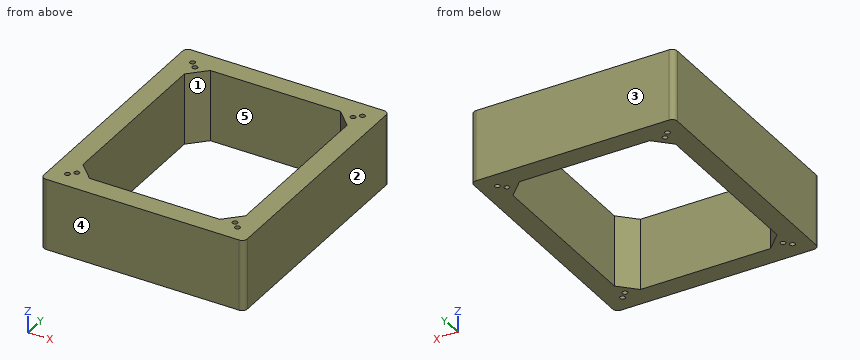
from build123d import *

# Parameters (mm, degrees)
F0_R     = 1.5875
F1_DEPTH = 44.45


with BuildPart() as f1:
    # F0 (on Top) → F1 (new body)
    with BuildSketch(Plane.XY):
        with BuildLine():
            Line((60.531797, 76.456334), (-60.118203, 76.456334))
            ThreePointArc((-60.118203, 76.456334), (-62.363267, 75.526399), (-63.293203, 73.281334))
            Line((-63.293203, 73.281334), (-63.293203, -72.768666))
            ThreePointArc((-63.293203, -72.768666), (-62.363267, -75.01373), (-60.118203, -75.943666))
            Line((-60.118203, -75.943666), (60.531797, -75.943666))
            ThreePointArc((60.531797, -75.943666), (62.776861, -75.01373), (63.706797, -72.768666))
            Line((63.706797, -72.768666), (63.706797, 73.281334))
            ThreePointArc((63.706797, 73.281334), (62.776861, 75.526399), (60.531797, 76.456334))
        make_face()
        with BuildLine():
            ThreePointArc((-56.943203, 66.931334), (-56.013267, 69.176399), (-53.768203, 70.106334))
            Line((-53.768203, 70.106334), (54.181797, 70.106334))
            ThreePointArc((54.181797, 70.106334), (56.426861, 69.176399), (57.356797, 66.931334))
            Line((57.356797, 66.931334), (57.356797, -66.418666))
            ThreePointArc((57.356797, -66.418666), (56.426861, -68.66373), (54.181797, -69.593666))
            Line((54.181797, -69.593666), (-53.768203, -69.593666))
            ThreePointArc((-53.768203, -69.593666), (-56.013267, -68.66373), (-56.943203, -66.418666))
            Line((-56.943203, -66.418666), (-56.943203, 66.931334))
        make_face(mode=Mode.SUBTRACT)
        with BuildLine():
            Line((54.181797, 70.106334), (-53.768203, 70.106334))
            ThreePointArc((-53.768203, 70.106334), (-56.013267, 69.176399), (-56.943203, 66.931334))
            Line((-56.943203, 66.931334), (-56.943203, -66.418666))
            ThreePointArc((-56.943203, -66.418666), (-56.013267, -68.66373), (-53.768203, -69.593666))
            Line((-53.768203, -69.593666), (54.181797, -69.593666))
            ThreePointArc((54.181797, -69.593666), (56.426861, -68.66373), (57.356797, -66.418666))
            Line((57.356797, -66.418666), (57.356797, 66.931334))
            ThreePointArc((57.356797, 66.931334), (56.426861, 69.176399), (54.181797, 70.106334))
        make_face()
        with Locations((-52.834257, -65.484719)):
            Circle(F0_R, mode=Mode.SUBTRACT)
        with BuildLine():
            ThreePointArc((-48.268948, 63.640233), (-47.847518, 63.727175), (-47.418203, 63.756334))
            Line((-47.418203, 63.756334), (-40.433203, 63.756334))
            Line((-40.433203, 63.756334), (40.846797, 63.756334))
            Line((40.846797, 63.756334), (47.831797, 63.756334))
            ThreePointArc((47.831797, 63.756334), (48.261112, 63.727175), (48.682541, 63.640233))
            ThreePointArc((48.682541, 63.640233), (50.321889, 63.738981), (51.171406, 62.333443))
            ThreePointArc((51.171406, 62.333443), (51.099604, 61.861412), (50.890695, 61.432079))
            ThreePointArc((50.890695, 61.432079), (50.977637, 61.01065), (51.006797, 60.581334))
            Line((51.006797, 60.581334), (51.006797, 53.596334))
            Line((51.006797, 53.596334), (51.006797, -53.083666))
            Line((51.006797, -53.083666), (51.006797, -60.698242))
            ThreePointArc((51.006797, -60.698242), (51.000133, -60.882306), (50.980177, -61.065405))
            ThreePointArc((50.980177, -61.065405), (51.122856, -61.431175), (51.171406, -61.820774))
            ThreePointArc((51.171406, -61.820774), (50.39662, -63.184465), (48.828536, -63.217046))
            ThreePointArc((48.828536, -63.217046), (48.645437, -63.237002), (48.461374, -63.243666))
            Line((48.461374, -63.243666), (40.846797, -63.243666))
            Line((40.846797, -63.243666), (-40.433203, -63.243666))
            Line((-40.433203, -63.243666), (-47.418203, -63.243666))
            ThreePointArc((-47.418203, -63.243666), (-47.847518, -63.214506), (-48.268948, -63.127564))
            ThreePointArc((-48.268948, -63.127564), (-50.292844, -62.943306), (-50.477102, -60.91941))
            ThreePointArc((-50.477102, -60.91941), (-50.564044, -60.497981), (-50.593203, -60.068666))
            Line((-50.593203, -60.068666), (-50.593203, -53.083666))
            Line((-50.593203, -53.083666), (-50.593203, 53.596334))
            Line((-50.593203, 53.596334), (-50.593203, 60.581334))
            ThreePointArc((-50.593203, 60.581334), (-50.564044, 61.01065), (-50.477102, 61.432079))
            ThreePointArc((-50.477102, 61.432079), (-50.292844, 63.455975), (-48.268948, 63.640233))
        make_face(mode=Mode.SUBTRACT)
        with Locations((53.24785, -65.484719)):
            Circle(F0_R, mode=Mode.SUBTRACT)
        with Locations((-52.834257, 65.997388)):
            Circle(F0_R, mode=Mode.SUBTRACT)
        with Locations((53.24785, 65.997388)):
            Circle(F0_R, mode=Mode.SUBTRACT)
        with BuildLine():
            Line((-40.433203, 63.756334), (-47.418203, 63.756334))
            ThreePointArc((-47.418203, 63.756334), (-47.847518, 63.727175), (-48.268948, 63.640233))
            ThreePointArc((-48.268948, 63.640233), (-47.764774, 63.071427), (-47.582812, 62.333443))
            ThreePointArc((-47.582812, 62.333443), (-48.69828, 60.817745), (-50.477102, 61.432079))
            ThreePointArc((-50.477102, 61.432079), (-50.564044, 61.01065), (-50.593203, 60.581334))
            Line((-50.593203, 60.581334), (-50.593203, 53.596334))
            Line((-50.593203, 53.596334), (-40.433203, 63.756334))
        make_face()
        with BuildLine():
            Line((47.831797, 63.756334), (40.846797, 63.756334))
            Line((40.846797, 63.756334), (51.006797, 53.596334))
            Line((51.006797, 53.596334), (51.006797, 60.581334))
            ThreePointArc((51.006797, 60.581334), (50.977637, 61.01065), (50.890695, 61.432079))
            ThreePointArc((50.890695, 61.432079), (48.461374, 61.210911), (48.682541, 63.640233))
            ThreePointArc((48.682541, 63.640233), (48.261112, 63.727175), (47.831797, 63.756334))
        make_face()
        with BuildLine():
            Line((51.006797, -60.698242), (51.006797, -53.083666))
            Line((51.006797, -53.083666), (40.846797, -63.243666))
            Line((40.846797, -63.243666), (48.461374, -63.243666))
            ThreePointArc((48.461374, -63.243666), (48.645437, -63.237002), (48.828536, -63.217046))
            ThreePointArc((48.828536, -63.217046), (48.461374, -60.698242), (50.980177, -61.065405))
            ThreePointArc((50.980177, -61.065405), (51.000133, -60.882306), (51.006797, -60.698242))
        make_face()
        with BuildLine():
            Line((-40.433203, -63.243666), (-50.593203, -53.083666))
            Line((-50.593203, -53.083666), (-50.593203, -60.068666))
            ThreePointArc((-50.593203, -60.068666), (-50.564044, -60.497981), (-50.477102, -60.91941))
            ThreePointArc((-50.477102, -60.91941), (-48.69828, -60.305076), (-47.582812, -61.820774))
            ThreePointArc((-47.582812, -61.820774), (-47.764774, -62.558758), (-48.268948, -63.127564))
            ThreePointArc((-48.268948, -63.127564), (-47.847518, -63.214506), (-47.418203, -63.243666))
            Line((-47.418203, -63.243666), (-40.433203, -63.243666))
        make_face()
    extrude(amount=F1_DEPTH)


solid = f1.part
The model under review builds one solid part; all positions refer to its coordinate system, in mm. Face numbers are marked on the shaded views. A direction names the side the tool comes from. Give positions to 0.01 mm unless a question says otherwise; leave off trailing zeros. Order: outer loops, then holes, each group sorted by start corner. A loop starts at its lowest first (then second) coordinate and runs counter-clockwise, first axis right, second up. Notation, with made-up numbers: M 64.25,66 L 109.25,66 A20 cw 109.25,84 Z; hole C 73.25,15 d1. An arc over 180 degrees is marked long. One line per question, with ' | ' between items. Start each with the question number.
1) Consider section B-B, the plane x = 15.5. Give the boundary of the cut face in (y, z).
2) Wall thickness on L1, parallel to X at y = -28.5, z = 16; L2, parallel to Y at x = -19.5, z = 39; L3, parallel to Y at x = 45, z = 7.5: over which ranges is each line inside the solid? List them lowest first. Write a range as from..to.
3) Consider section A-A, the plane y = 23.5. Give the boundary of the cut face in (x, z).
4) Mouldability with a two-part tool opening along X and no side actions: class the marked faces 1, 2 and 3 as pulls with the +X half, pulls with the -X half, needs draft (parallel to the pull), parting line crosses it, or undercut.
5) For the marked faces 4 and 5, list the 3-axis set-ups (+Z, -Z, +X, -X, +Y, -Y) from which the entire face can be reached by the end or side of a thin tool; tool diameter is ignored.
6) Consider section C-C, the plane z = 25. State how many separate pieces and enclosed holes the cut face has, then the cut area to 3 significant figures.
Found:
1) outline: M -75.94,0 L -63.24,0 L -63.24,44.45 L -75.94,44.45 Z; M 63.76,0 L 76.46,0 L 76.46,44.45 L 63.76,44.45 Z
2) L1: x = -63.29..-50.59, 51.01..63.71 | L2: y = -75.94..-63.24, 63.76..76.46 | L3: y = -75.94..-59.09, 59.6..76.46
3) outline: M -63.29,0 L -50.59,0 L -50.59,44.45 L -63.29,44.45 Z; M 51.01,0 L 63.71,0 L 63.71,44.45 L 51.01,44.45 Z
4) face 1: undercut | face 2: pulls with the +X half | face 3: needs draft
5) face 4: +Z, -Z, +X, -X, -Y | face 5: +Z, -Z
6) separate pieces: 1 | enclosed holes: 9 | area: 6,590 mm²
